from build123d import *

# Parameters (mm, degrees)
SKETCH1_R               = 7.9375
BOSS_EXTRUDE1_DEPTH     = 7.112
SKETCH2_R               = 5.715
BOSS_EXTRUDE2_DEPTH     = 7.112
BOSS_EXTRUDE3_DEPTH     = 10.16
SKETCH4_R               = 1.5
CUT_EXTRUDE1_DEPTH      = 50.53
CUT_EXTRUDE2_DEPTH      = 23.219226796
BOSS_EXTRUDE5_DEPTH     = 10.16
CUT_EXTRUDE3_DEPTH      = 4.180773204
CUT_EXTRUDE3_DEPTH_BACK = 23.219226796
CUT_EXTRUDE5_DEPTH      = 23.219226896
CUT_EXTRUDE6_DEPTH      = 10.16
BOSS_EXTRUDE6_DEPTH     = 10.16
CUT_EXTRUDE7_DEPTH      = 4.180773304
CUT_EXTRUDE7_DEPTH_BACK = 23.219226896
BOSS_EXTRUDE7_START     = -16.899912
BOSS_EXTRUDE7_DEPTH     = 14.76137


with BuildPart() as part:
    # Sketch1 → Boss-Extrude1 (new body)
    with BuildSketch(Plane.XY):
        with BuildLine():
            ThreePointArc((9.519226796, 15.24), (12.7, 0), (9.519226796, -15.24))
            Line((9.519226796, -15.24), (-9.519226796, -15.24))
            ThreePointArc((-9.519226796, -15.24), (-12.7, 0), (-9.519226796, 15.24))
            Line((-9.519226796, 15.24), (9.519226796, 15.24))
        make_face()
        Circle(SKETCH1_R, mode=Mode.SUBTRACT)
        Polygon((5.362175987, 24.765), (9.519226796, 15.24), (-9.519226796, 15.24), (-5.362175987, 24.765), align=None)
        Polygon((-9.519226796, -15.24), (9.519226796, -15.24), (5.362175987, -24.765), (-5.362175987, -24.765), align=None)
    extrude(amount=BOSS_EXTRUDE1_DEPTH)

    # Sketch2 → Boss-Extrude2 (add)
    with BuildSketch(Plane(origin=(0, 0, 0), x_dir=(-1, 0, 0), z_dir=(0, 0, -1))):
        with BuildLine():
            Line((9.519226796, -15.24), (-9.519226796, -15.24))
            ThreePointArc((-9.519226796, -15.24), (-12.7, 0), (-9.519226796, 15.24))
            Line((-9.519226796, 15.24), (9.519226796, 15.24))
            ThreePointArc((9.519226796, 15.24), (12.7, 0), (9.519226796, -15.24))
        make_face()
        Circle(SKETCH2_R, mode=Mode.SUBTRACT)
    extrude(amount=BOSS_EXTRUDE2_DEPTH)

    # Sketch3 → Boss-Extrude3 (add)
    with BuildSketch(Plane.XY.offset(7.112)):
        Polygon((5.362175987, 24.765), (9.519226796, 15.24), (-9.519226796, 15.24), (-5.362175987, 24.765), align=None)
        Polygon((5.362175987, -24.765), (9.519226796, -15.24), (-9.519226796, -15.24), (-5.362175987, -24.765), align=None)
    extrude(amount=BOSS_EXTRUDE3_DEPTH)

    # Sketch4 → Cut-Extrude1 (cut, through all)
    with BuildSketch(Plane(origin=(0, 24.765, 0), x_dir=(1, 0, 0), z_dir=(0, 1, 0))):
        with Locations((0, -13.756694386)):
            Circle(SKETCH4_R)
    extrude(amount=-CUT_EXTRUDE1_DEPTH, mode=Mode.SUBTRACT)

    # Sketch5 → Cut-Extrude2 (cut, through all)
    with BuildSketch(Plane.ZY.offset(9.519226796)):
        Polygon((0, 15.24), (10.224694386, 24.765), (0, 24.765), align=None)
        Polygon((17.272, 15.24), (17.272, 18.26514), (9.652, 18.26514), (7.112, 15.72514), (7.112, 15.24), align=None)
    extrude(amount=-CUT_EXTRUDE2_DEPTH, mode=Mode.SUBTRACT)

    # Sketch6 → Boss-Extrude5 (add)
    with BuildSketch(Plane.XY.offset(7.112)):
        with BuildLine():
            Line((-7.612509174, 15.24), (-9.519226796, 15.24))
            ThreePointArc((-9.519226796, 15.24), (-10.875837369, 11.647902093), (-11.864005337, 7.9375))
            Line((-11.864005337, 7.9375), (-11.102005337, 7.9375))
            Line((-11.102005337, 7.9375), (-7.612509174, 15.24))
        make_face()
        Polygon((-9.307494341, 15.72514), (-9.519226796, 15.24), (-7.612509174, 15.24), (-7.380685255, 15.72514), align=None)
        Polygon((-8.198947459, 18.26514), (-9.307494341, 15.72514), (-7.380685255, 15.72514), (-6.166947459, 18.26514), align=None)
        Polygon((8.198947459, 18.26514), (6.166947459, 18.26514), (7.380685255, 15.72514), (9.307494341, 15.72514), align=None)
        Polygon((7.380685255, 15.72514), (7.612509174, 15.24), (9.519226796, 15.24), (9.307494341, 15.72514), align=None)
        with BuildLine():
            Line((9.519226796, 15.24), (7.612509174, 15.24))
            Line((7.612509174, 15.24), (11.102005337, 7.9375))
            Line((11.102005337, 7.9375), (11.864005337, 7.9375))
            ThreePointArc((11.864005337, 7.9375), (10.875837369, 11.647902093), (9.519226796, 15.24))
        make_face()
    extrude(amount=BOSS_EXTRUDE5_DEPTH)

    # Sketch7 → Cut-Extrude3 (cut, two sides)
    with BuildSketch(Plane.ZY.offset(9.519226796)) as cut_extrude3_sk:
        Polygon((7.112, 7.9375), (17.272, 15.24), (17.272, 7.9375), align=None)
        with BuildLine():
            Line((8.403818024, 11.307371095), (11.919117111, 13.833992314))
            ThreePointArc((11.919117111, 13.833992314), (12.103221267, 14.39329083), (11.627299087, 14.74))
            Line((11.627299087, 14.74), (8.112, 14.74))
            ThreePointArc((8.112, 14.74), (7.758446609, 14.593553391), (7.612, 14.24))
            Line((7.612, 14.24), (7.612, 11.713378781))
            ThreePointArc((7.612, 11.713378781), (7.883865185, 11.268457995), (8.403818024, 11.307371095))
        make_face()
    extrude(amount=CUT_EXTRUDE3_DEPTH, mode=Mode.SUBTRACT)
    extrude(cut_extrude3_sk.sketch, amount=-CUT_EXTRUDE3_DEPTH_BACK, mode=Mode.SUBTRACT)

    # Sketch9 → Cut-Extrude5 (cut, through all)
    with BuildSketch(Plane.ZY.offset(9.519226796)):
        Polygon((0, -24.765), (10.224694386, -24.765), (0, -15.24), align=None)
    extrude(amount=-CUT_EXTRUDE5_DEPTH, mode=Mode.SUBTRACT)

    # Sketch8 → Cut-Extrude6 (cut)
    with BuildSketch(Plane.XY.offset(17.272)):
        Polygon((7.612509174, -15.24), (-7.612509174, -15.24), (-6.166947459, -18.26514), (6.166947459, -18.26514), align=None)
    extrude(amount=-CUT_EXTRUDE6_DEPTH, mode=Mode.SUBTRACT)

    # Sketch10 → Boss-Extrude6 (add)
    with BuildSketch(Plane.XY.offset(7.112)):
        with BuildLine():
            Line((-9.519226796, -15.24), (-7.612509174, -15.24))
            Line((-7.612509174, -15.24), (-11.102005337, -7.9375))
            Line((-11.102005337, -7.9375), (-11.864005337, -7.9375))
            ThreePointArc((-11.864005337, -7.9375), (-10.875837369, -11.647902093), (-9.519226796, -15.24))
        make_face()
        with BuildLine():
            Line((7.612509174, -15.24), (9.519226796, -15.24))
            ThreePointArc((9.519226796, -15.24), (10.875837369, -11.647902093), (11.864005337, -7.9375))
            Line((11.864005337, -7.9375), (11.102005337, -7.9375))
            Line((11.102005337, -7.9375), (7.612509174, -15.24))
        make_face()
    extrude(amount=BOSS_EXTRUDE6_DEPTH)

    # Sketch11 → Cut-Extrude7 (cut, two sides)
    with BuildSketch(Plane.ZY.offset(9.519226796)) as cut_extrude7_sk:
        Polygon((17.272, -15.24), (17.272, -7.9375), (7.112, -7.9375), align=None)
        with BuildLine():
            ThreePointArc((8.112, -14.74), (7.758446609, -14.593553391), (7.612, -14.24))
            Line((7.612, -14.24), (7.612, -11.713378781))
            ThreePointArc((7.612, -11.713378781), (7.883865185, -11.268457995), (8.403818024, -11.307371095))
            Line((8.403818024, -11.307371095), (11.919117111, -13.833992314))
            ThreePointArc((11.919117111, -13.833992314), (12.103221267, -14.39329083), (11.627299087, -14.74))
            Line((11.627299087, -14.74), (8.112, -14.74))
        make_face()
    extrude(amount=CUT_EXTRUDE7_DEPTH, mode=Mode.SUBTRACT)
    extrude(cut_extrude7_sk.sketch, amount=-CUT_EXTRUDE7_DEPTH_BACK, mode=Mode.SUBTRACT)

    # Sketch12 → Boss-Extrude7 (add)
    with BuildSketch(Plane.ZY.offset(9.519226796).offset(BOSS_EXTRUDE7_START)):
        Polygon((7.112, -18.26514), (7.112, -15.72514), (9.652, -18.26514), align=None)
    extrude(amount=BOSS_EXTRUDE7_DEPTH)


solid = part.part
Source: CAD feature listing. Evaluate the final solid. Frame: model axes, mm. A direction names the side the tool comes from. Round coordinates to 2 decimals unless told otherwise and drop trailing zeros. Loops run counter-clockwise (first coordinate to the right, second up) from the corner with the lowest first, then second, coordinate; pieces in that order, holes last. Notation, with made-up numbers: (-20, 74) - (5, 74) arc R17 cw to (5, 97) - close; hole circle Ø11 at (-15.5, -23). An arc over 180 degrees is marked (long way). Write item = value, one per line. Start each with the question number.
(1) Ray query, line 1 along X through (y, z) = (0, 5.5); line 2 along Y through (x, z) = (2, -1); line 3 along Y through (x, z) = (0, -2) (3 decimals). Return the intervals inside material, ascending. Write a range as from..to.
(2) Section query C-C, the plane z = -1. Output: boundary loops of the cut face in (x, y) (3 decimals), plus the area to 3 significant figures.
(3) Section query D-D, the plane y = 21. Output: boundary loops of the cut face in (x, z).
(4) Section query B-B, the plane x = 0. State how many separate pieces and enclosed holes the cut face has, plus the area to 3 significant figures.
(5) Section query A-A, the plane y = 0. Output: boundary loops of the cut face in (x, z) (1 decimal), plus the area to 3 significant figures.
(6) Pin query (flat end, axial travel): pin 1 (5 mm diameter, centred on y = 8, z = 3, fed in from +X); pin 2 (0.9 mm diameter, centred on x = -8.5, z = 9.5, fed in from +Y); pin 3 (1.5 mm diameter, centred on y = -11.5, z = -3.5, fed in from +X). Return the tip coordinate at first contact, or that it passes through.
(7) Pull-direction query (X, two-part tool) for faces 1 (the face through (3.4, -5.2, 0)), 2 (the face through (-10, -12.1, 12.9)); classes: +X half, -X half, draft (parallel to the pull), parting line (faces both ways), or undercut.
(8) Set-up query: faces 3 (the face through (8.3, 0.2, 7.112)), 4 (the face through (-9, -13, 7.612)), 5 (the face through (10, -12.1, 12.9)). Return all of +Z, -Z, +X, -X, +Y, -Y with unobstructed straight access to the full face (end or side cutting, diameter ignored); none if empty.
Conclusion:
q1.line_1 = -12.7..-7.94, 7.94..12.7
q1.line_2 = -15.24..-5.35, 5.35..15.24
q1.line_3 = -15.24..-5.715, 5.715..15.24
q2.outline = (-9.519, -15.24) - (9.519, -15.24) arc R38.1 ccw to (9.519, 15.24) - (-9.519, 15.24) arc R38.1 ccw to start; hole circle Ø11.43 at (0, 0)
q2.area = 608 mm2
q3.outline = (-7.01, 6.18) - (7.01, 6.18) - (7.01, 17.27) - (-7.01, 17.27) - close; hole circle Ø3 at (0, 13.76)
q4.separate_pieces = 4
q4.enclosed_holes = 0
q4.area = 377 mm2
q5.outline = (-12.7, -7.1) - (-5.7, -7.1) - (-5.7, 0) - (-7.9, 0) - (-7.9, 7.1) - (-12.7, 7.1) - close; (5.7, -7.1) - (12.7, -7.1) - (12.7, 7.1) - (7.9, 7.1) - (7.9, 0) - (5.7, 0) - close
q5.area = 167 mm2
q6.pin_1 = 12.3
q6.pin_2 = 18.61
q6.pin_3 = 11.15
q7.face_1 = undercut
q7.face_2 = draft
q8.face_3 = +Z
q8.face_4 = +X, -X
q8.face_5 = +Z, +X, -X
